Design review of the part built by this model. Coordinates are the model's own, in mm. Coordinates: 2 decimals unless noted, no trailing zeros. Write each loop counter-clockwise with the first axis right and the second up, starting at its lowest first coordinate (ties: lowest second). Pieces come first, ordered by that corner, then holes. Notation, with made-up numbers: M -4,53.25 L 28,53.25 A27 ccw 28,78.25 Z; hole C 32,61 d11. An arc over 180 degrees is marked long. One line per question, with ' | ' between items.
from build123d import *

# Parameters (mm, degrees)
F0_R     = 123.825
F1_DEPTH = 3.175
F2_R     = 22.225
F3_DEPTH = 25.4
F4_R     = 12.7
F5_DEPTH = 50.8


with BuildPart() as f1:
    # F0 (on Front) → F1 (new body, symmetric)
    with BuildSketch(Plane.XZ):
        Circle(F0_R)
    extrude(amount=F1_DEPTH, both=True)

    # F2 (on face) → F3 (join)
    with BuildSketch(Plane.XZ.offset(3.175)):
        Circle(F2_R)
    extrude(amount=F3_DEPTH)

    # F4 (on face) → F5 (cut, symmetric)
    with BuildSketch(Plane.XZ.offset(28.575)):
        Circle(F4_R)
    extrude(amount=F5_DEPTH, both=True, mode=Mode.SUBTRACT)


solid = f1.part
1. To check wall thickness, follow line 1 along Z through (x, y) = (0, -20) (3 decimals); line 2 along Y through (x, z) = (-90.5, -60) (3 decimals); line 3 along X through (y, z) = (1, -7.5). State the ranges of each line that lie inside material, in increasing order. Write a range as [from, to].
Answer sheet:
line 1: [-22.225, -12.7], [12.7, 22.225] | line 2: [-3.175, 3.175] | line 3: [-123.6, -10.25], [10.25, 123.6]
2. Take a section at C-C (y = -6). Write out the cut boundary in (x, z) (3 decimals).
Answer sheet:
outline: C 0,0 d44.45; hole C 0,0 d25.4
3. Take a section at B-B (z = 0). Write out the cut boundary in (x, y) (3 decimals).
Answer sheet:
outline: M -123.825,-3.175 L -22.225,-3.175 L -22.225,-28.575 L -12.7,-28.575 L -12.7,3.175 L -123.825,3.175 Z; M 12.7,-28.575 L 22.225,-28.575 L 22.225,-3.175 L 123.825,-3.175 L 123.825,3.175 L 12.7,3.175 Z
4. Draft analysis for pull direction Z (two halves, no side actions). For faces 1 (the face through (21.199, -15.697, 6.676)), 2 (the face through (10, -28.575, -10)), 3 (the face through (-2.75, -12.92, -12.4)), state which applies: pulls with the +Z half, pulls with the -Z half, needs draft (parallel to the pull), parting line crosses it, or undercut.
Answer sheet:
face 1: parting line crosses it | face 2: needs draft | face 3: undercut
5. Insertion check: pin 1 Ø5 at (x, y) = (-15, -18.5) entering from -Z; pin 2 Ø1 at (x, y) = (-8, -7.5) entering from -Z; pin 3 Ø12 at (y, z) = (-8, 51) entering from -X. Each pin has a flat end and moves straight along its axis. Give the tip position at first contact, or say it passes through.
Answer sheet:
pin 1: z = -18.38 | pin 2: z = -20.92 | pin 3: x = -114.38
6. Take a section at D-D (z = -109). Write out the cut boundary in (x, y) (3 decimals).
Answer sheet:
outline: M -58.751,-3.175 L 58.751,-3.175 L 58.751,3.175 L -58.751,3.175 Z
7. Take a section at A-A (x = 0). Write out the cut boundary in (y, z) (3 decimals).
Answer sheet:
outline: M -28.575,-22.225 L -3.175,-22.225 L -3.175,-123.825 L 3.175,-123.825 L 3.175,-12.7 L -28.575,-12.7 Z; M -28.575,12.7 L 3.175,12.7 L 3.175,123.825 L -3.175,123.825 L -3.175,22.225 L -28.575,22.225 Z
